Part model, mm, in its own coordinate system. A direction names the side the tool comes from. Give positions to 0.01 mm unless a question says otherwise; leave off trailing zeros. Order: outer loops, then holes, each group sorted by start corner. A loop starts at its lowest first (then second) coordinate and runs counter-clockwise, first axis right, second up. Notation, with made-up numbers: M -37,-40 L -3,-40 A34 ccw -3,-9 Z; hole C -39.5,23.5 d2. An arc over 180 degrees is marked long. Return JSON: item names as keys, results as strings.
from build123d import *

# Parameters (mm, degrees)
ESQUISSE1_R        = 4.85
BOSS_EXTRU_1_DEPTH = 8
ESQUISSE2_R        = 3.35
BOSS_EXTRU_2_DEPTH = 2


with BuildPart() as part:
    # Esquisse1 → Boss.-Extru.1 (new body)
    with BuildSketch(Plane.XY):
        with Locations((0, 1)):
            Circle(ESQUISSE1_R)
        with BuildLine():
            Line((-1.5, 2), (1.5, 2))
            ThreePointArc((1.5, 2), (0, -2.5), (-1.5, 2))
        make_face(mode=Mode.SUBTRACT)
    extrude(amount=BOSS_EXTRU_1_DEPTH)

    # Esquisse2 → Boss.-Extru.2 (add)
    with BuildSketch(Plane.XY.offset(8)):
        Circle(ESQUISSE2_R)
    extrude(amount=BOSS_EXTRU_2_DEPTH)


solid = part.part
Q1. Two-plate mould, pull along Y, no slides. Class faces 1 (the flat face through (0, 0, 8)), 2 (the flat face through (0, 4, 8)), 3 (the cylindrical face through (-3.347, 0.147, 8.986)): +Y half, -Y half, draft (parallel to the pull), parting line (faces both ways), or undercut.
Established:
{"face 1": "undercut", "face 2": "draft", "face 3": "parting line"}
Q2. Probe line 1 along Y through (x, z) = (0, 3); line 2 along Z through (x, y) = (-0.25, 3.75); line 3 along Z through (x, y) = (1.75, 1). List the from-to ranges inside material, lowest first.
Established:
{"line 1": "y = -3.85 to -2.5, 2 to 5.85", "line 2": "z = 0 to 8", "line 3": "z = 8 to 10"}
Q3. Band-saw the part on C-C (y = 0.25). Give the cut face in (x, z).
Established:
{"outline": "M -4.79,0 L -2.49,0 L -2.49,8 L 2.49,8 L 2.49,0 L 4.79,0 L 4.79,8 L 3.34,8 L 3.34,10 L -3.34,10 L -3.34,8 L -4.79,8 Z"}
Q4. Band-saw the part on B-B (z = 4.25). Give the cut face in (x, y).
Established:
{"outline": "C 0,1 d9.7; hole M -1.5,2 A2.5 ccw long 1.5,2 Z"}
Q5. Pin check, flat tips, straight feed: pin 1 (3.5 mm diameter, centred on x = 0, y = 0.5, fed in from -Z); pin 2 (3 mm diameter, centred on x = 0, y = 0, fed in from -Z); pin 3 (1.5 mm diameter, centred on x = -2.5, z = 3.5, fed in from +Y); pin 4 (1.5 mm diameter, centred on x = 2.5, z = 3.5, fed in from -Y). Stop position of each tip, or through.
Established:
{"pin 1": "stops at z = 0", "pin 2": "stops at z = 8", "pin 3": "stops at y = 5.52", "pin 4": "stops at y = -3.52"}
Q6. 3-axis set-ups, long thin cutter, end or side, ignore diameter. For faces 4 (the flat face through (0, 3, 0)), 5 (the flat face through (0, 2, 4)): which of +Z, -Z, +X, -X, +Y, -Y reach the whole face in a straight line?
Established:
{"face 4": "-Z, +X, -X, +Y, -Y", "face 5": "-Z"}
Q7. Band-saw the part on D-D (z = 8.25). Give the cut face in (x, y).
Established:
{"outline": "C 0,0 d6.7"}
Q8. Band-saw the part on A-A (x = 0). Give the cut face in (y, z).
Established:
{"outline": "M -3.85,0 L -2.5,0 L -2.5,8 L 2,8 L 2,0 L 5.85,0 L 5.85,8 L 3.35,8 L 3.35,10 L -3.35,10 L -3.35,8 L -3.85,8 Z"}
